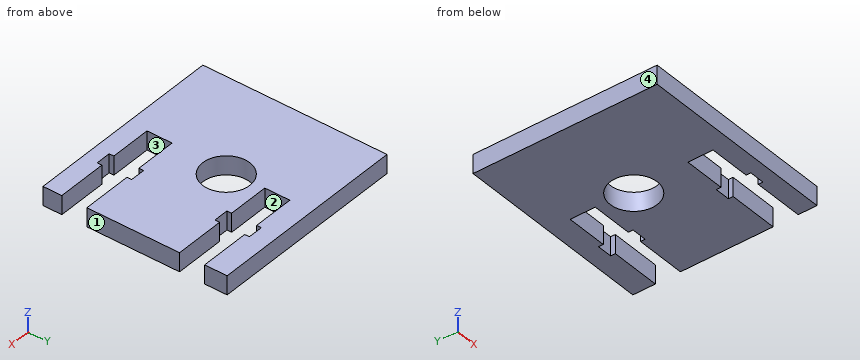
```python
from build123d import *

# Parameters (mm, degrees)
SKETCH1_W           = 31.901767955
SKETCH1_H           = 28.791004307
BOSS_EXTRUDE2_DEPTH = 3
SKETCH3_R           = 3.75
CUT_EXTRUDE1_DEPTH  = 33
CUT_EXTRUDE2_DEPTH  = 33
SKETCH6_W           = 31.901767955
SKETCH6_H           = 0.59
BOSS_EXTRUDE3_DEPTH = 3


with BuildPart() as part:
    # Sketch1 → Boss-Extrude2 (new body)
    with BuildSketch(Plane.XY):
        with Locations((13.594756215, 69.164541294)):
            Rectangle(SKETCH1_W, SKETCH1_H)
    extrude(amount=BOSS_EXTRUDE2_DEPTH)

    # Sketch3 → Cut-Extrude1 (cut)
    with BuildSketch(Plane(origin=(0, 0, 0), x_dir=(-1, 0, 0), z_dir=(0, 0, -1))):
        with Locations((-13.297916625, 71.016762707)):
            Circle(SKETCH3_R)
    extrude(amount=-CUT_EXTRUDE1_DEPTH, mode=Mode.SUBTRACT)

    # Sketch5 → Cut-Extrude2 (cut)
    with BuildSketch(Plane.XY.offset(3)):
        Polygon((29.545640192, 76.560043447), (21.555740858, 76.560043447), (21.555740858, 75.810043447), (19.155740858, 75.810043447), (19.155740858, 76.560043447), (12.545640192, 76.560043447), (12.545640192, 80.560043447), (19.155740858, 80.560043447), (19.155740858, 81.310043447), (21.555740858, 81.310043447), (21.555740858, 80.560043447), (29.545640192, 80.560043447), align=None)
        Polygon((29.545640192, 57.76903914), (29.545640192, 61.76903914), (21.555740858, 61.76903914), (21.555740858, 62.51903914), (19.155740858, 62.51903914), (19.155740858, 61.76903914), (12.545640192, 61.76903914), (12.545640192, 57.76903914), (19.155740858, 57.76903914), (19.155740858, 57.01903914), (21.555740858, 57.01903914), (21.555740858, 57.76903914), align=None)
    extrude(amount=-CUT_EXTRUDE2_DEPTH, mode=Mode.SUBTRACT)

    # Sketch6 → Boss-Extrude3 (add)
    with BuildSketch(Plane.XY.offset(3)):
        with Locations((13.594756215, 83.855043447)):
            Rectangle(SKETCH6_W, SKETCH6_H)
    extrude(amount=-BOSS_EXTRUDE3_DEPTH)


solid = part.part
```
For this review, take the finished solid that the model builds, in its own axes (mm). Face numbers are marked on the shaded views. A direction names the side the tool comes from. Give positions to 0.01 mm unless a question says otherwise; leave off trailing zeros. Write each loop counter-clockwise with the first axis right and the second up, starting at its lowest first coordinate (ties: lowest second). Pieces come first, ordered by that corner, then holes. Notation, with made-up numbers: M -15.5,39.5 L 27.5,39.5 A33 ccw 27.5,71.5 Z; hole C 83.5,74 d11. An arc over 180 degrees is marked long. Answer as CSV lines item,"result".
1. Consider section B-B, the plane x = 11.5. Write out the cut boundary in (y, z), then the cut area to 3 significant figures.
Findings:
outline,"M 54.77,0 L 67.73,0 L 67.73,3 L 54.77,3 Z; M 74.31,0 L 84.15,0 L 84.15,3 L 74.31,3 Z"
area,"68.4 mm2"
2. Consider section D-D, the plane x = 27.5. Write out the cut boundary in (y, z).
Findings:
outline,"M 54.77,0 L 57.77,0 L 57.77,3 L 54.77,3 Z; M 61.77,0 L 76.56,0 L 76.56,3 L 61.77,3 Z; M 80.56,0 L 84.15,0 L 84.15,3 L 80.56,3 Z"
3. For the marked faces 3 and 4, list the 3-axis set-ups (+Z, -Z, +X, -X, +Y, -Y) from which the entire face can be reached by the end or side of a thin tool; tool diameter is ignored.
Findings:
face 3,"+Z, -Z, +X"
face 4,"+Z, -Z, -X, +Y, -Y"
4. Draft analysis for pull direction Y (two halves, no side actions). For the marked faces 1 and 2, state which applies: +Y half, -Y half, draft (parallel to the pull), parting line (faces both ways), or undercut.
Findings:
face 1,"draft"
face 2,"undercut"
5. Wall thickness on line 1 (Y direction, x = 26, z = 2.5); line 2 (Y direction, x = 21.5, z = 0.6); line 3 (Y direction, x = 13.5, z = 1.1): over which ranges is each line inside the solid? List them lowest first.
Findings:
line 1,"y = 54.77 to 57.77, 61.77 to 76.56, 80.56 to 84.15"
line 2,"y = 54.77 to 57.02, 62.52 to 75.81, 81.31 to 84.15"
line 3,"y = 54.77 to 57.77, 61.77 to 67.27, 74.76 to 76.56, 80.56 to 84.15"
6. Consider section A-A, the plane x = 21. Write out the cut boundary in (y, z).
Findings:
outline,"M 54.77,0 L 57.02,0 L 57.02,3 L 54.77,3 Z; M 62.52,0 L 75.81,0 L 75.81,3 L 62.52,3 Z; M 81.31,0 L 84.15,0 L 84.15,3 L 81.31,3 Z"
7. For pin 1 (0.9 mm diameter, centred on y = 79.5, z = 2, fed in from +X), flat-tipped, find the tip position at first contact; note if it passes through.
Findings:
pin 1,"stops at x = 12.55"
